Model file for the job. Use its own axes, mm. Give positions to 0.01 mm unless a question says otherwise; leave off trailing zeros. Order: outer loops, then holes, each group sorted by start corner. A loop starts at its lowest first (then second) coordinate and runs counter-clockwise, first axis right, second up. Notation, with made-up numbers: (-21, 84) - (-14, 84) arc R23 ccw to (-14, 117) - close; hole circle Ø3 at (42, 68). An arc over 180 degrees is marked (long way). Use CSV: the item, a comma, the result in double quotes. Start each with the question number.
(1) Band-saw the part on B-B, the plane y = 146.1. Give the cut face in (x, z), then the cut area to 3 significant figures.
(2) Drop a flat-ended pin along its axis: pin 1 Ø1 at (x, z) = (85.5, -0.5) entering from -Y. Give the stop position or say it passes through.
(3) Band-saw the part on D-D, the plane y = 144. Give the cut face in (x, z).
(4) Pull direction Z, two halves, no side cores. Call faces 1 (the flat face through (85.1, 147, 2)), 2 (the cylindrical face through (86.418, 149.517, -0.759)), 3 (the cylindrical face through (86.418, 144.365, -0.228)): +Z half, -Z half, draft (parallel to the pull), parting line (faces both ways), or undercut.
(5) Band-saw the part on C-C, the plane x = 86.4. Give the cut face in (y, z), then the cut area to 3 significant figures.
(6) Probe L1, parallel to Y at x = 86.85, z = 0; L2, parallel to Z at x = 86.7, y = 146.1; L3, parallel to Y at x = 87.05, z = 0.75. List the from-to ranges inside material, lowest first.
(7) Band-saw the part on A-A, the plane z = 0. Give the cut face in (x, y), then the cut area to 3 significant figures.
from build123d import *

# Parameters (mm, degrees)
SKETCH15_W   = 26
SKETCH15_H   = 35
SKETCH16_W   = 26
SKETCH16_H   = 17.5
SCALE1_SCALE = 0.1


with BuildPart() as part:
    # Sketch15 → Revolve1 (revolve)
    with BuildSketch(Plane.XY, mode=Mode.PRIVATE) as revolve1_sk:
        with Locations((864, 1478.5)):
            Rectangle(SKETCH15_W, SKETCH15_H)
    revolve(revolve1_sk.sketch.rotate(Axis((851, 1461, 0), (1, 0, 0)), 90), axis=Axis((851, 1461, 0), (1, 0, 0)))

    # Sketch16 → Cut-Revolve1 (revolve, cut)
    with BuildSketch(Plane.XY, mode=Mode.PRIVATE) as cut_revolve1_sk:
        with Locations((864, 1469.75)):
            Rectangle(SKETCH16_W, SKETCH16_H)
    revolve(cut_revolve1_sk.sketch.rotate(Axis((851, 1461, 0), (1, 0, 0)), 90), axis=Axis((851, 1461, 0), (1, 0, 0)), mode=Mode.SUBTRACT)


with BuildPart() as part_1:
    # Scale1: scaled about (0, 0, 0)
    add(part.part.scale(SCALE1_SCALE))


solid = part_1.part
Answer block:
1,outline,"(85.1, -3.5) - (87.7, -3.5) - (87.7, -1.75) - (85.1, -1.75) - close; (85.1, 1.75) - (87.7, 1.75) - (87.7, 3.5) - (85.1, 3.5) - close"
1,area,"9.10 mm2"
2,pin 1,"stops at y = 142.6"
3,outline,"(85.1, -2.8) - (87.7, -2.8) - (87.7, 2.8) - (85.1, 2.8) - close"
4,face 1,"draft"
4,face 2,"parting line"
4,face 3,"undercut"
5,outline,"circle Ø7 at (146.1, 0); hole circle Ø3.5 at (146.1, 0)"
5,area,"28.9 mm2"
6,L1,"y = 142.6 to 144.35, 147.85 to 149.6"
6,L2,"z = -3.5 to -1.75, 1.75 to 3.5"
6,L3,"y = 142.68 to 144.52, 147.68 to 149.52"
7,outline,"(85.1, 142.6) - (87.7, 142.6) - (87.7, 144.35) - (85.1, 144.35) - close; (85.1, 147.85) - (87.7, 147.85) - (87.7, 149.6) - (85.1, 149.6) - close"
7,area,"9.10 mm2"
